Verification items for the finished model (mm, model axes). A direction names the side the tool comes from. Coordinates: 2 decimals unless noted, no trailing zeros. Order: outer loops, then holes, each group sorted by start corner. A loop starts at its lowest first (then second) coordinate and runs counter-clockwise, first axis right, second up. Notation, with made-up numbers: (11.5, -39.75) -> (56.5, -39.75) arc R25 cw to (56.5, -7.75) -> close; hole circle Ø7 at (44, 32.5). An arc over 180 degrees is marked (long way). Answer as CSV lines item,"result".
```python
from build123d import *

# Parameters (mm, degrees)
F1_DEPTH = 23
F3_DEPTH = 25
F4_W     = 30
F4_H     = 12
F5_DEPTH = 3


with BuildPart() as f1:
    # F0 (on Top) → F1 (new body)
    with BuildSketch(Plane.XY):
        with BuildLine():
            Line((-101.79164, -46.223918), (-41.771353, -46.223918))
            Line((-41.771353, -46.223918), (-40.522749, -49.773918))
            Line((-40.522749, -49.773918), (-38.79164, -49.773918))
            Line((-38.79164, -49.773918), (-38.79164, -46.673918))
            Line((-38.79164, -46.673918), (-39.29164, -46.673918))
            Line((-39.29164, -46.673918), (-39.29164, -44.573918))
            Line((-39.29164, -44.573918), (-38.79164, -44.573918))
            Line((-38.79164, -44.573918), (-37.79164, -44.573918))
            Line((-37.79164, -44.573918), (-37.79164, -43.573918))
            Line((-37.79164, -43.573918), (-39.79164, -43.573918))
            Line((-39.79164, -43.573918), (-39.79164, -48.838682))
            Line((-39.79164, -48.838682), (-41.29164, -44.573918))
            Line((-41.29164, -44.573918), (-101.79164, -44.573918))
            ThreePointArc((-101.79164, -44.573918), (-104.241978, -48.572254), (-99.567025, -48.940578))
            ThreePointArc((-99.567025, -48.940578), (-99.561923, -48.926017), (-99.565678, -48.911052))
            Line((-99.565678, -48.911052), (-100.36651, -47.566828))
            ThreePointArc((-100.36651, -47.566828), (-100.565096, -47.47099), (-100.731146, -47.616072))
            ThreePointArc((-100.731146, -47.616072), (-102.666674, -47.990488), (-101.79164, -46.223918))
        make_face()
    extrude(amount=F1_DEPTH)

    # F2 (on face) → F3 (cut)
    with BuildSketch(Plane(origin=(0, 0, 0), x_dir=(1, 0, 0), z_dir=(0, 0, -1))):
        Polygon((-39.385125, 49.773918), (-38.79164, 47.239013), (-38.79164, 49.773918), align=None)
    extrude(amount=-F3_DEPTH, mode=Mode.SUBTRACT)

    # F4 (on face) → F5 (join)
    with BuildSketch(Plane.XZ.offset(46.223918)):
        with Locations((-71.771353, 12)):
            Rectangle(F4_W, F4_H)
    extrude(amount=F5_DEPTH)


solid = f1.part
```
Item 1: Section check C-C, the plane x = -44. Record the boundary of the cut face in (y, z), plus the area to 4 significant figures.
Answer list:
outline,"(-46.22, 0) -> (-44.57, 0) -> (-44.57, 23) -> (-46.22, 23) -> close"
area,"37.95 mm2"
Item 2: Section check B-B, the plane y = -45.25. Record the boundary of the cut face in (x, z).
Answer list:
outline,"(-103.6, 0) -> (-41.05, 0) -> (-41.05, 23) -> (-103.6, 23) -> close; (-39.79, 0) -> (-39.29, 0) -> (-39.29, 23) -> (-39.79, 23) -> close"
Item 3: Tool access check on faces 1 (the flat face through (-39, -44.574, 11)), 2 (the flat face through (-72, -48, 18)), 3 (the flat face through (-71, -44.574, 11)), 4 (the flat face through (-99.96, -48.25, 11.34)). Record the directions out of +Z, -Z, +X, -X, +Y, -Y that give a thin tool (end or side, any length) a straight path to the whole face; none if there is none.
Answer list:
face 1,"+Z, -Z, +X"
face 2,"+Z, -Y"
face 3,"+Z, -Z, -X, +Y"
face 4,"+Z, -Z"
Item 4: Release check for a two-part mould opening along Y. For faces 5 (the flat face through (-40, -49.774, 11)), 6 (the flat face through (-39.292, -46, 11)), 7 (the flat face through (-86.771, -48, 12)), 8 (the cylindrical face through (-104.277, -48.502, 11.339)) record: +Y half, -Y half, draft (parallel to the pull), parting line (faces both ways), or undercut.
Answer list:
face 5,"-Y half"
face 6,"undercut"
face 7,"draft"
face 8,"parting line"
Item 5: Section check A-A, the plane x = -80.5. Record the boundary of the cut face in (y, z).
Answer list:
outline,"(-49.22, 6) -> (-46.22, 6) -> (-46.22, 0) -> (-44.57, 0) -> (-44.57, 23) -> (-46.22, 23) -> (-46.22, 18) -> (-49.22, 18) -> close"
Item 6: Thickness scan on line 1 (Y direction, x = -86, z = 13); line 2 (Y direction, x = -69.5, z = 5.5); line 3 (X direction, y = -45.25, z = 7.5). Record the ranges inside material, lowest first.
Answer list:
line 1,"-49.22 to -44.57"
line 2,"-46.22 to -44.57"
line 3,"-103.6 to -41.05, -39.79 to -39.29"
Item 7: Depth check by flat-ended pin: pin 1 Ø1.5 at (x, z) = (-97, 11.5) entering from +Y; pin 2 Ø1.5 at (y, z) = (-46, 18.5) entering from +X; pin 3 Ø0.6 at (x, z) = (-40, 7) entering from -Y. Enter the tip coordinate at first touch or a pass-through.
Answer list:
pin 1,"y = -44.57"
pin 2,"x = -38.79"
pin 3,"y = -49.77"
